from build123d import *

# Parameters (mm, degrees)
SKETCH1_W              = 30
SKETCH1_H              = 17
BOSS_EXTRUDE1_DEPTH    = 6
SKETCH234_W            = 10
SKETCH234_H            = 6
BOSS_EXTRUDE234_DEPTH  = 6
FILLET134_R            = 1
SKETCH2341_W           = 10
SKETCH2341_H           = 6
BOSS_EXTRUDE2341_DEPTH = 6
FILLET1341_R           = 1
M3_CLEARANCE_HOLE1_D   = 3.2
FILLET1342_R           = 5


with BuildPart() as part:
    # Sketch1 → Boss-Extrude1 (new body)
    with BuildSketch(Plane(origin=(0, 0, 0), x_dir=(1, 0, 0), z_dir=(0, 1, 0))):
        with Locations((15, 8.5)):
            Rectangle(SKETCH1_W, SKETCH1_H)
    extrude(amount=BOSS_EXTRUDE1_DEPTH)

    # Sketch234 → Boss-Extrude234 (add)
    with BuildSketch(Plane(origin=(4.232221392, 0, 0), x_dir=(1, 0, 0), z_dir=(0, 0, 1))):
        with Locations((0.767778608, 3)):
            Rectangle(SKETCH234_W, SKETCH234_H)
    extrude(amount=BOSS_EXTRUDE234_DEPTH)

    # Fillet134
    fillet134_edges = [part.edges().sort_by_distance(p)[0] for p in [
        (0, 3, 6),
        (10, 3, 6),
    ]]
    fillet(fillet134_edges, radius=FILLET134_R)

    # Sketch2341 → Boss-Extrude2341 (add)
    with BuildSketch(Plane(origin=(24.232221392, 0, 0), x_dir=(1, 0, 0), z_dir=(0, 0, 1))):
        with Locations((0.767778608, 3)):
            Rectangle(SKETCH2341_W, SKETCH2341_H)
    extrude(amount=BOSS_EXTRUDE2341_DEPTH)

    # Fillet1341
    fillet1341_edges = [part.edges().sort_by_distance(p)[0] for p in [
        (30, 3, 6),
        (20, 3, 6),
    ]]
    fillet(fillet1341_edges, radius=FILLET1341_R)

    # M3 Clearance Hole1 (through all)
    with Locations(Plane(origin=(0, 6, 0), x_dir=(1, 0, 0), z_dir=(0, 1, 0))):
        with Locations((5, 12), (25, 12)):
            Hole(M3_CLEARANCE_HOLE1_D / 2)

    # Fillet1342
    fillet1342_edges = [part.edges().sort_by_distance(p)[0] for p in [
        (0, 3, -17),
        (30, 3, -17),
    ]]
    fillet(fillet1342_edges, radius=FILLET1342_R)


solid = part.part
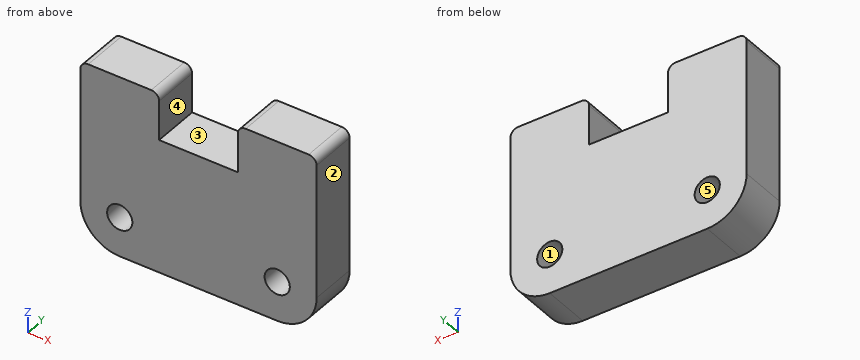
Geometry: final body of the model. Coordinates: model frame, mm. Face numbers are marked on the shaded views. A direction names the side the tool comes from. Give positions to 0.01 mm unless a question says otherwise; leave off trailing zeros. Order: outer loops, then holes, each group sorted by start corner. A loop starts at its lowest first (then second) coordinate and runs counter-clockwise, first axis right, second up. Notation, with made-up numbers: (41.5, 77) -> (94.5, 77) arc R18 ccw to (94.5, 103) -> close; hole circle Ø3 at (75, 26.25). An arc over 180 degrees is marked (long way). Answer as a JSON object with one key per item and string values.
Q1. Access query for the marked faces 4 and 5. Directions: +Z, -Z, +X, -X, +Y, -Y. A direction counts if a zero-diameter tool reaches every point of the face in a straight line with its end or side. Return the directions, or none.
Entries:
{"face 4": "+Z, +Y, -Y", "face 5": "+Y, -Y"}
Q2. First-contact query: pin 1 (1.9 mm diameter, centred on x = 5, z = -12, fed in from +Y); pin 2 (1.8 mm diameter, centred on x = 16, y = 1.5, fed in from +Z). Flat tips, straight axial feed; report the tip coordinate or a pass-through.
Entries:
{"pin 1": "passes through", "pin 2": "stops at z = 0"}
Q3. Section B-B (x = 24.5). Output: boundary loops of the cut face in (y, z), plus the area to 3 significant figures.
Entries:
{"outline": "(0, -17) -> (6, -17) -> (6, -13.52) -> (0, -13.52) -> close; (0, -10.48) -> (6, -10.48) -> (6, 6) -> (0, 6) -> close", "area": "120 mm^2"}
Q4. Section C-C (x = 11.5). Output: boundary loops of the cut face in (y, z).
Entries:
{"outline": "(0, -17) -> (6, -17) -> (6, 0) -> (0, 0) -> close"}
Q5. Section A-A (y = 2.35). Output: boundary loops of the cut face in (x, z), plus the area to 3 significant figures.
Entries:
{"outline": "(0, -12) arc R5 ccw to (5, -17) -> (25, -17) arc R5 ccw to (30, -12) -> (30, 5) arc R1 ccw to (29, 6) -> (21, 6) arc R1 ccw to (20, 5) -> (20, 0) -> (10, 0) -> (10, 5) arc R1 ccw to (9, 6) -> (1, 6) arc R1 ccw to (0, 5) -> close; hole circle Ø3.2 at (5, -12); hole circle Ø3.2 at (25, -12)", "area": "602 mm^2"}
Q6. Material intervals for probe 1 along X at (y, z) = (4.1, -12); probe 2 along Z at (x, y) = (25, 3.85); probe 3 along X at (y, z) = (1.5, 3.5), sorted ascending.
Entries:
{"probe 1": "x = 0 to 3.4, 6.6 to 23.4, 26.6 to 30", "probe 2": "z = -17 to -13.6, -10.4 to 6", "probe 3": "x = 0 to 10, 20 to 30"}
Q7. Draft query along Z for the marked faces 1, 2 and 3. Return one class per face: released by +Z, released by -Z, zero draft, split by the parting line, or undercut.
Entries:
{"face 1": "undercut", "face 2": "zero draft", "face 3": "released by +Z"}
